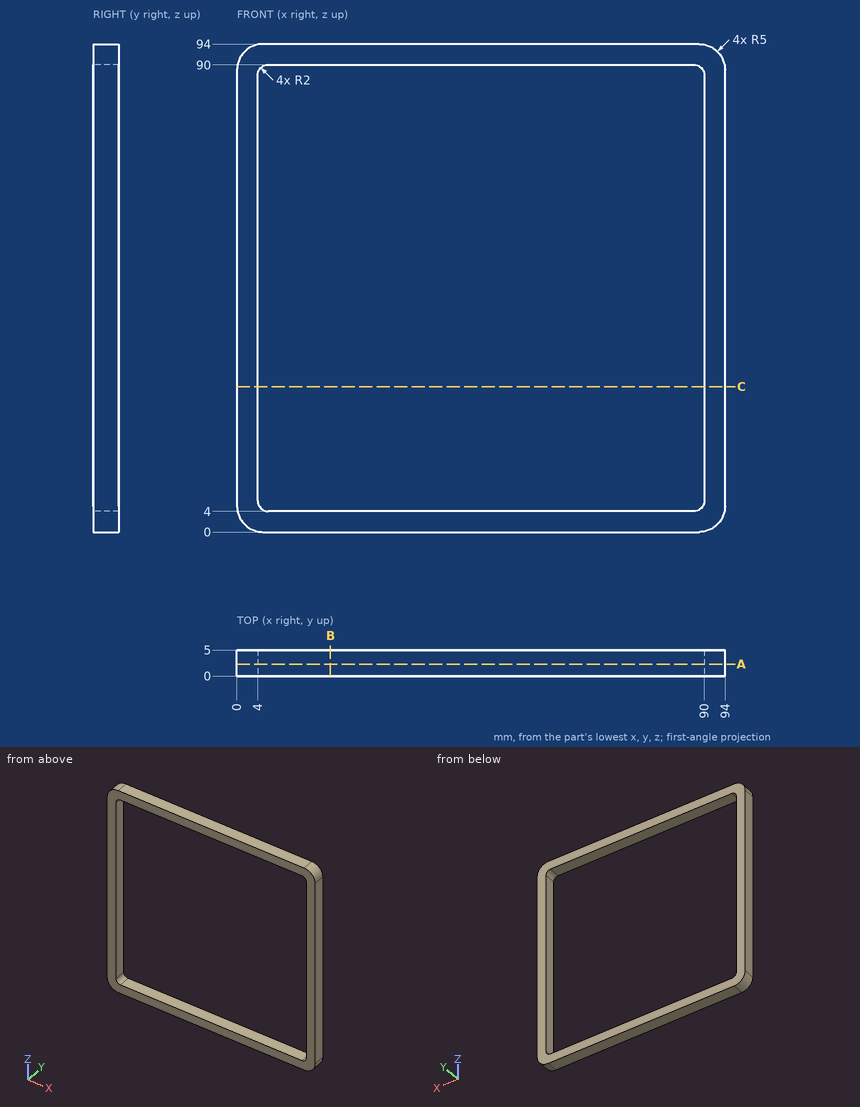
Could you check a few things on this drawing? It's one solid part, dimensions in mm from its lowest x, y, z. Coordinates: 2 decimals unless noted, no trailing zeros. Order: outer loops, then holes, each group sorted by start corner. A loop starts at its lowest first (then second) coordinate and runs counter-clockwise, first axis right, second up. Notation, with made-up numbers: M -11.75,37.5 L 33.25,37.5 A7 ccw 33.25,50.5 Z; hole C -5,70 d4. An arc over 180 degrees is marked long. Answer as a JSON object with one key per item and string values. Group by question number.
(1) I need wall thicknesses on probe 1 along Z at (x, y) = (66, 3.65). Which ranges of the line are inside material? Lowest first, please.
(2) Suppose I cut it at A-A, the plane y = 2.3. Please give me the cut outline in (x, z).
(3) Suppose I cut it at C-C, the plane z = 28. Please give me the cut outline in (x, y).
(4) Suppose I cut it at B-B, the plane x = 18. Please give me the cut outline in (y, z), then the cut area to 3 significant figures.
Values found:
{
 "1": {"probe 1": "z = 0 to 4, 90 to 94"},
 "2": {"outline": "M 0,5 A5 ccw 5,0 L 89,0 A5 ccw 94,5 L 94,89 A5 ccw 89,94 L 5,94 A5 ccw 0,89 Z; hole M 4,6 A2 ccw 6,4 L 88,4 A2 ccw 90,6 L 90,88 A2 ccw 88,90 L 6,90 A2 ccw 4,88 Z"},
 "3": {"outline": "M 0,0 L 4,0 L 4,5 L 0,5 Z; M 90,0 L 94,0 L 94,5 L 90,5 Z"},
 "4": {"outline": "M 0,0 L 5,0 L 5,4 L 0,4 Z; M 0,90 L 5,90 L 5,94 L 0,94 Z", "area": "40.0 mm^2"}
}
